from build123d import *

# Parameters (mm, degrees)
PAD_DEPTH    = 3.5
SKETCH001_R  = 1.6
POCKET_DEPTH = 20.001


with BuildPart() as part:
    # Sketch → Pad (new body, symmetric)
    with BuildSketch(Plane.XY):
        Polygon((-20, 14.5), (0, 14.5), (0, -17), (-4, -17), (-4, 0), (-20, 0), (-20, 4), (-4, 4), (-4, 10.5), (-20, 10.5), align=None)
    extrude(amount=PAD_DEPTH, both=True)

    # Sketch001 → Pocket (cut, through all)
    with BuildSketch(Plane.YZ):
        with Locations((-3.5, 0)):
            Circle(SKETCH001_R)
        with Locations((-13.5, 0)):
            Circle(SKETCH001_R)
    extrude(amount=-POCKET_DEPTH, mode=Mode.SUBTRACT)


solid = part.part
Here's how the part is built. I have some questions about the finished solid (model axes, mm). A direction names the side the tool comes from. Round coordinates to 2 decimals unless told otherwise and drop trailing zeros. Order: outer loops, then holes, each group sorted by start corner. A loop starts at its lowest first (then second) coordinate and runs counter-clockwise, first axis right, second up. Notation, with made-up numbers: (-34.5, 27.5) -> (-15.5, 27.5) arc R28 cw to (-15.5, 66.5) -> close; hole circle Ø1 at (78, 0). An arc over 180 degrees is marked (long way). Return JSON: item names as keys, results as strings.
Q1. For pin 1 Ø2 at (y, z) = (9, 0.5) entering from +X; pin 2 Ø2 at (x, z) = (-11, 1.5) entering from -Y; pin 3 Ø3 at (y, z) = (8, -1.5) entering from -X, each with a flat end and sliding along its axis, tell me the tip position at first contact or that it passes through.
Filled sheet:
{"pin 1": "stops at x = 0", "pin 2": "stops at y = 0", "pin 3": "stops at x = -4"}
Q2. If we section it at A-A on x = -9.5: List the corners of the cut face in (y, z) for me, plus the area to 3 significant figures.
Filled sheet:
{"outline": "(0, -3.5) -> (4, -3.5) -> (4, 3.5) -> (0, 3.5) -> close; (10.5, -3.5) -> (14.5, -3.5) -> (14.5, 3.5) -> (10.5, 3.5) -> close", "area": "56.0 mm^2"}
Q3. Which directions (+Z, -Z, +X, -X, +Y, -Y) give clear straight access to the entire face, cutting with the end or side of a thin tool? Please do faces 4 (the flat face through (-20, 12, 0)), 5 (the flat face through (-12, 4, 0)), 6 (the flat face through (-4, -9, 0)).
Filled sheet:
{"face 4": "+Z, -Z, -X, +Y, -Y", "face 5": "+Z, -Z, -X", "face 6": "+Z, -Z, -X, -Y"}
Q4. If we section it at C-C on y = -13.5: List the corners of the cut face in (x, z) for me, plus the area to 3 significant figures.
Filled sheet:
{"outline": "(-4, -3.5) -> (0, -3.5) -> (0, -1.6) -> (-4, -1.6) -> close; (-4, 1.6) -> (0, 1.6) -> (0, 3.5) -> (-4, 3.5) -> close", "area": "15.2 mm^2"}
Q5. I need wall thicknesses on line 1 along Z through (x, y) = (-2.5, -13.5); line 2 along Y through (x, z) = (-18.5, -1); line 3 along X through (y, z) = (-1, -1). Which ranges of each line are inside material? Lowest first, please. Write a range as from..to.
Filled sheet:
{"line 1": "z = -3.5..-1.6, 1.6..3.5", "line 2": "y = 0..4, 10.5..14.5", "line 3": "x = -4..0"}
Q6. If we section it at D-D on z = -2.25: List the corners of the cut face in (x, y) for me, plus the area to 3 significant figures.
Filled sheet:
{"outline": "(-20, 0) -> (-4, 0) -> (-4, -17) -> (0, -17) -> (0, 14.5) -> (-20, 14.5) -> (-20, 10.5) -> (-4, 10.5) -> (-4, 4) -> (-20, 4) -> close", "area": "254 mm^2"}
Q7. If we section it at B-B on z = 0: List the corners of the cut face in (x, y) for me, plus the area to 3 significant figures.
Filled sheet:
{"outline": "(-20, 0) -> (-4, 0) -> (-4, -1.9) -> (0, -1.9) -> (0, 14.5) -> (-20, 14.5) -> (-20, 10.5) -> (-4, 10.5) -> (-4, 4) -> (-20, 4) -> close; (-4, -17) -> (0, -17) -> (0, -15.1) -> (-4, -15.1) -> close; (-4, -11.9) -> (0, -11.9) -> (0, -5.1) -> (-4, -5.1) -> close", "area": "228 mm^2"}
Q8. If we mould it in two halves opening along Z, with no side actions, what happens to faces 1 (the flat face through (-5, 2, -3.5)), 2 (the cylindrical face through (-1.97, -2.02, -0.61)), 3 (the flat face through (-12, 10.5, 0))? For each: released by +Z, released by -Z, zero draft, split by the parting line, or undercut.
Filled sheet:
{"face 1": "released by -Z", "face 2": "undercut", "face 3": "zero draft"}
